Work out the finished part from the listing and answer in its coordinate system (mm). A direction names the side the tool comes from. Round coordinates to 2 decimals unless told otherwise and drop trailing zeros. Write each loop counter-clockwise with the first axis right and the second up, starting at its lowest first coordinate (ties: lowest second). Pieces come first, ordered by that corner, then holes. Notation, with made-up numbers: (56.25, 33.5) -> (66.25, 33.5) arc R25 cw to (66.25, 53.5) -> close; hole circle Ø9 at (59, 56). An arc over 180 degrees is marked (long way). One line per question, with ' | ' between items. Start each with the question number.
```python
from build123d import *

# Parameters (mm, degrees)
SKETCH1_W           = 360
SKETCH1_H           = 80
BOSS_EXTRUDE1_DEPTH = 12
CUT_EXTRUDE1_REACH  = 186.781
SKETCH2_R           = 2.5
CUT_EXTRUDE2_DEPTH  = 8
CUT_EXTRUDE3_DEPTH  = 6.5
LPATTERN1_COUNT     = 4
LPATTERN1_PITCH     = 90
SKETCH7_R           = 12
CUT_EXTRUDE4_DEPTH  = 8
CUT_EXTRUDE5_REACH  = 186.564
SKETCH8_R           = 11


with BuildPart() as part:
    # Sketch1 → Boss-Extrude1 (new body)
    with BuildSketch(Plane.XY):
        Rectangle(SKETCH1_W, SKETCH1_H)
    extrude(amount=BOSS_EXTRUDE1_DEPTH)

    # Sketch2 → Cut-Extrude1 (cut, up to next)
    with BuildSketch(Plane.XY.offset(12), mode=Mode.PRIVATE) as cut_extrude1_sk1:
        with Locations((-135, 32)):
            Circle(SKETCH2_R)
    cut_extrude1_tool1 = extrude(cut_extrude1_sk1.sketch, amount=-CUT_EXTRUDE1_REACH, mode=Mode.PRIVATE) & part.part
    cut_extrude1 = cut_extrude1_tool1.solids().sort_by_distance((-135, 32, 12))[0]
    add(cut_extrude1, mode=Mode.SUBTRACT)

    # Sketch4 → Cut-Extrude2 (cut)
    with BuildSketch(Plane(origin=(-23.391380574, 111.176150639, 0), x_dir=(-1, 0, 0), z_dir=(0, 0, -1))):
        with BuildLine():
            Line((107.608619426, -137.176150639), (115.608619426, -137.176150639))
            ThreePointArc((115.608619426, -137.176150639), (117.608619426, -139.176150639), (115.608619426, -141.176150639))
            Line((115.608619426, -141.176150639), (107.608619426, -141.176150639))
            ThreePointArc((107.608619426, -141.176150639), (105.608619426, -139.176150639), (107.608619426, -137.176150639))
        make_face()
    cut_extrude2 = extrude(amount=-CUT_EXTRUDE2_DEPTH, mode=Mode.SUBTRACT)

    # Sketch6 → Cut-Extrude3 (cut)
    with BuildSketch(Plane(origin=(-23.391380574, 111.176150639, 0), x_dir=(-1, 0, 0), z_dir=(0, 0, -1))):
        with BuildLine():
            Line((114.108619426, -134.176150639), (114.108619426, -164.82997736))
            ThreePointArc((114.108619426, -164.82997736), (111.608619426, -167.32997736), (109.108619426, -164.82997736))
            Line((109.108619426, -164.82997736), (109.108619426, -134.176150639))
            ThreePointArc((109.108619426, -134.176150639), (111.608619426, -131.676150639), (114.108619426, -134.176150639))
        make_face()
    cut_extrude3 = extrude(amount=-CUT_EXTRUDE3_DEPTH, mode=Mode.SUBTRACT)

    # LPattern1: Cut-Extrude1, Cut-Extrude2, Cut-Extrude3 ×4
    with Locations(*[(i * LPATTERN1_PITCH, 0, 0) for i in range(1, LPATTERN1_COUNT)]):
        add(cut_extrude1, mode=Mode.SUBTRACT)
        add(cut_extrude2, mode=Mode.SUBTRACT)
        add(cut_extrude3, mode=Mode.SUBTRACT)

    # Sketch7 → Cut-Extrude4 (cut)
    with BuildSketch(Plane(origin=(0, 0, 0), x_dir=(-1, 0, 0), z_dir=(0, 0, -1))):
        with Locations((0, -10.5)):
            Circle(SKETCH7_R)
    extrude(amount=-CUT_EXTRUDE4_DEPTH, mode=Mode.SUBTRACT)

    # Sketch8 → Cut-Extrude5 (cut, up to next)
    with BuildSketch(Plane(origin=(0, 0, 8), x_dir=(-1, 0, 0), z_dir=(0, 0, -1)), mode=Mode.PRIVATE) as cut_extrude5_sk1:
        with Locations((0, -10.5)):
            Circle(SKETCH8_R)
    cut_extrude5_tool1 = extrude(cut_extrude5_sk1.sketch, amount=-CUT_EXTRUDE5_REACH, mode=Mode.PRIVATE) & part.part
    add(cut_extrude5_tool1.solids().sort_by_distance((0, -10.5, 8))[0], mode=Mode.SUBTRACT)


solid = part.part
```
(1) For faces 4 (the flat face through (-180, -1, 6)), 5 (the flat face through (-137.5, -35, 3)), 6 (the flat face through (45, -26, 7)), determine the directions among +Z, -Z, +X, -X, +Y, -Y from which every point of the face is accessible in a straight line to the end or side of a thin tool.
(2) The mould has two halves that part along X. Classify faces 1 (the flat face through (-42.5, -35, 3)), 2 (the flat face through (180, -1, 6)), 3 (the flat face through (-3, -40, 6)): +X half, -X half, draft (parallel to the pull), parting line (faces both ways), or undercut.
(3) Consider L1, parallel to Y at x = 0, z = 2; L2, parallel to Y at x = -138.5, z = 3.25; L3, parallel to X at y = 33, z = 10. Determine where each line is inside the solid, lowest interval first.
(4) Given pin 1 Ø6.5 at (x, z) = (46.5, 4.5) entering from -Y; pin 2 Ø1.2 at (x, y) = (-136, -28.5) entering from -Z, each flat-ended and moving along its own axis, determine where each tip first touches the part or whether it passes through.
(5) A cutting plane is placed at B-B, the plane y = -10.5. Determine the outline of the cut face in (x, z), then the cut area to 3 significant figures.
(6) A cutting plane is placed at C-C, the plane z = 2. Count the separate pieces of the cut face and the enclosed holes in it, then the cut area to 3 significant figures.
(7) A cutting plane is placed at A-A, the plane x = 0. Determine the outline of the cut face in (y, z).
Returned:
1) face 4: +Z, -Z, -X, +Y, -Y | face 5: -Z, -Y | face 6: -Z
2) face 1: undercut | face 2: +X half | face 3: draft
3) L1: -40 to -22.5, 1.5 to 40 | L2: -40 to -30, -26 to 40 | L3: -180 to -137.29, -132.71 to -47.29, -42.71 to 42.71, 47.29 to 132.71, 137.29 to 180
4) pin 1: y = -40 | pin 2: z = 8
5) outline: (-180, 0) -> (-12, 0) -> (-12, 8) -> (-11, 8) -> (-11, 12) -> (-180, 12) -> close; (11, 8) -> (12, 8) -> (12, 0) -> (180, 0) -> (180, 12) -> (11, 12) -> close | area: 4,040 mm2
6) separate pieces: 1 | enclosed holes: 5 | area: 27,800 mm2
7) outline: (-40, 0) -> (-22.5, 0) -> (-22.5, 8) -> (-21.5, 8) -> (-21.5, 12) -> (-40, 12) -> close; (0.5, 8) -> (1.5, 8) -> (1.5, 0) -> (40, 0) -> (40, 12) -> (0.5, 12) -> close
